Solid Edge part; units mm, degrees
sketch "Sketch1" plane through (0, 0, 0) normal (0, 0, 1) x (1, 0, 0)
  line L0 (12.5, 7.5) -> (12.5, -7.5)
  line L1 (12.5, -7.5) -> (7.5, -7.5)
  line L2 (7.5, -7.5) -> (7.5, 7.5)
  line L3 (7.5, 7.5) -> (12.5, 7.5)
extrude "Protrusion1" add sketch "Sketch1" along normal blind 13
sketch "Sketch2" plane through (12.5, 0, 6.5) normal (1, 0, 0) x (0, 1, 0)
  line L0 (-3.9, -1.3) -> (-3.9, 6.5)
  line L1 (-3.9, 6.5) -> (3.9, 6.5)
  line L2 (3.9, 6.5) -> (3.9, -1.3)
  line L3 (3.9, -1.3) -> (-3.9, -1.3)
extrude "ProtrusiónExtruida_2" add sketch "Sketch2" along normal blind 13
sketch "Sketch3" plane through (0, 0, 0) normal (0, 0, 1) x (1, 0, 0)
  line L0 (7.5, 7.5) -> (2.3647, 7.5)
  line L1 (7.5, 3.9043) -> (2.3647, 7.5)
  line L2 (7.5, 7.5) -> (7.5, 3.9043)
  line L3 (7.5, -3.9043) -> (2.3647, -7.5)
  line L4 (7.5, -7.5) -> (2.3647, -7.5)
  line L5 (7.5, -7.5) -> (7.5, -3.9043)
extrude "Protrusion2" add sketch "Sketch3" along normal up to vertex (13 mm away)
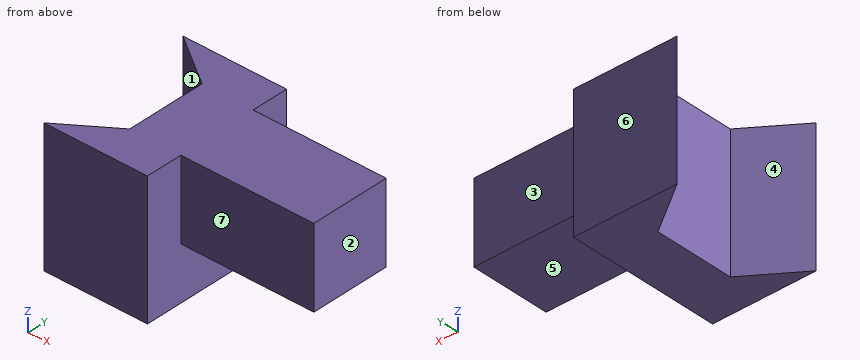
Here's how the part is built. I have some questions about the finished solid (model axes, mm). Face numbers are marked on the shaded views. A direction names the side the tool comes from. Coordinates: 2 decimals unless noted, no trailing zeros. Order: outer loops, then holes, each group sorted by start corner. A loop starts at its lowest first (then second) coordinate and runs counter-clockwise, first axis right, second up. Notation, with made-up numbers: (58, 51) - (66, 51) arc R26 ccw to (66, 84) - close; hole circle Ø8 at (15.5, 61.25). An arc over 180 degrees is marked (long way). Use CSV: the item, a comma, the result in double quotes. Start each with the question number.
1. Suppose I cut it at D-D on x = 20. List the corners of the cut face in (y, z) for me, then the cut area to 3 significant figures.
2. I'm going to push flat-ended pins straight in: pin 1 (2.5 mm diameter, centred on y = -0.5, z = 7.5, fed in from -X); pin 2 (3 mm diameter, centred on x = 17, z = 11, fed in from -Y); pin 3 (8.5 mm diameter, centred on x = 16.5, y = 0, fed in from -Z); pin 4 (1.5 mm diameter, centred on y = 3.5, z = 11, fed in from -X). Where does each tip first touch, or does it pass through?
3. Suppose I cut it at C-C on y = 1.5. List the corners of the cut face in (x, z) for me.
4. Suppose I cut it at B-B on z = 12. List the corners of the cut face in (x, y) for me.
5. Please list where these lines run through material, in increasing order: line 1 (Y direction, x = 15.75, z = 8.25); line 2 (X direction, y = 2, z = 9.75); line 3 (Z direction, x = 15, y = 3.75). Write a range as from..to.
6. Suppose I cut it at A-A on x = 4.5. List the corners of the cut face in (y, z) for me.
7. If we mould it in two halves opening along Y, with no side actions, what happens to the marked faces 4, 5, 6 and 7? For each: +Y half, -Y half, draft (parallel to the pull), parting line (faces both ways), or undercut.
8. For the marked faces 1, 2 and 3, which set-ups out of +Z, -Z, +X, -X, +Y, -Y let a thin tool reach every point of the face, with its end or its side?
Output:
1,outline,"(-3.9, 5.2) - (3.9, 5.2) - (3.9, 13) - (-3.9, 13) - close"
1,area,"60.8 mm2"
2,pin 1,"stops at x = 7.5"
2,pin 2,"stops at y = -3.9"
2,pin 3,"stops at z = 0"
2,pin 4,"stops at x = 7.01"
3,outline,"(7.5, 0) - (12.5, 0) - (12.5, 5.2) - (25.5, 5.2) - (25.5, 13) - (7.5, 13) - close"
4,outline,"(2.36, -7.5) - (12.5, -7.5) - (12.5, -3.9) - (25.5, -3.9) - (25.5, 3.9) - (12.5, 3.9) - (12.5, 7.5) - (2.36, 7.5) - (7.5, 3.9) - (7.5, -3.9) - close"
5,line 1,"y = -3.9..3.9"
5,line 2,"x = 7.5..25.5"
5,line 3,"z = 5.2..13"
6,outline,"(-7.5, 0) - (-6, 0) - (-6, 13) - (-7.5, 13) - close; (6, 0) - (7.5, 0) - (7.5, 13) - (6, 13) - close"
7,face 4,"undercut"
7,face 5,"draft"
7,face 6,"+Y half"
7,face 7,"-Y half"
8,face 1,"+Z, -Z, -X"
8,face 2,"+Z, -Z, +X, +Y, -Y"
8,face 3,"+Z, -Z, +X, +Y"
